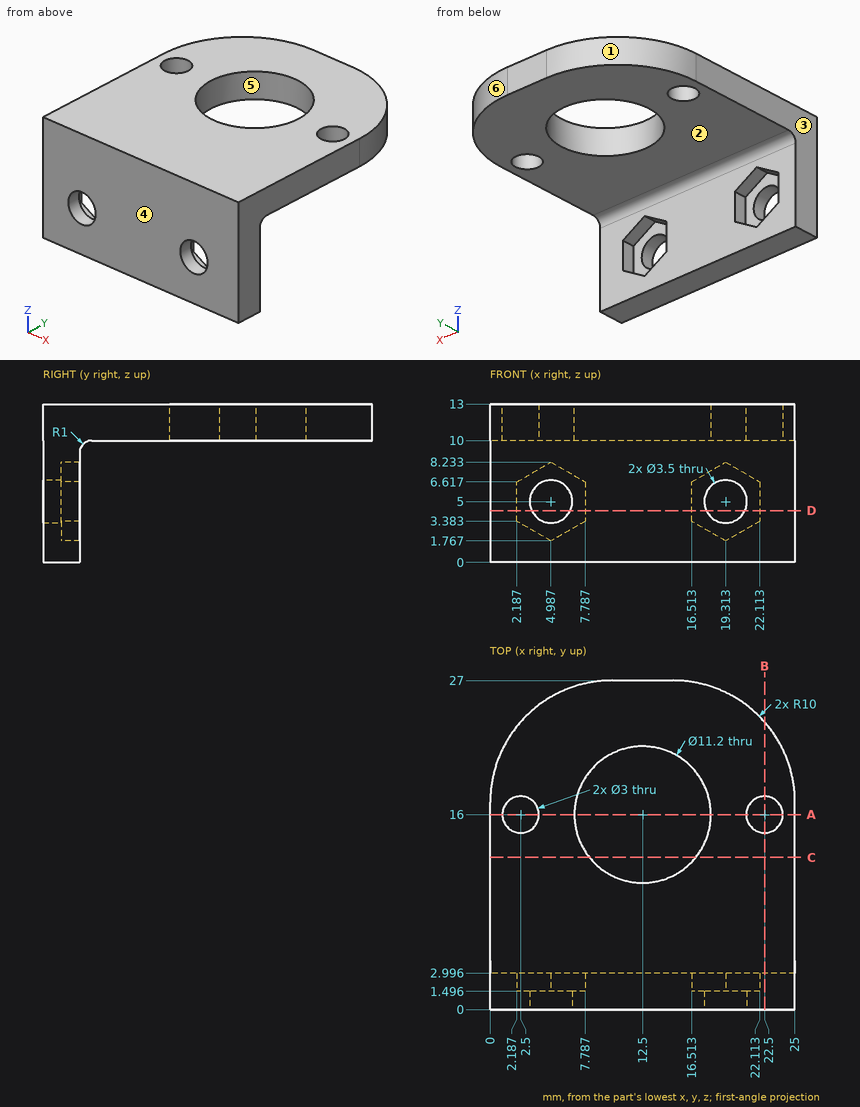
Could you check a few things on this drawing? It's one solid part, dimensions in mm from its lowest x, y, z. A direction names the side the tool comes from. Give positions to 0.01 mm unless a question says otherwise; leave off trailing zeros. Write each loop counter-clockwise with the first axis right and the second up, starting at its lowest first coordinate (ties: lowest second). Pieces come first, ordered by that corner, then holes.
(1) Imagine slicing it at B-B, the plane x = 22.5. Write out the boundary of the cut face in (y, z) (1 decimal).
Output values:
outline: (0, 0) - (3, 0) - (3, 9) arc R1 cw to (4, 10) - (14.5, 10) - (14.5, 13) - (0, 13) - close; (17.5, 10) - (23.6, 10) - (23.6, 13) - (17.5, 13) - close
(2) Imagine slicing it at A-A, the plane y = 16. Write out the boundary of the cut face in (x, z), and give its area (3 significant figures).
Output values:
outline: (0, 10) - (1, 10) - (1, 13) - (0, 13) - close; (4, 10) - (6.9, 10) - (6.9, 13) - (4, 13) - close; (18.1, 10) - (21, 10) - (21, 13) - (18.1, 13) - close; (24, 10) - (25, 10) - (25, 13) - (24, 13) - close
area: 23.4 mm2
(3) On a 3-axis mill with a long thin cutter (end or side, diameter ignored), from which of +Z, -Z, +X, -X, +Y, -Y can I reach the whole of each face in a straight line? I mean the marked faces 1 and 2. Say none if no direction works.
Output values:
face 1: +Z, -Z, -X, +Y
face 2: -Z, +X, -X, +Y
(4) Will these pins go through, and if not, where does the flat tip stop? pin 1 (1.7 mm diameter, centred on x = 18, z = 6, fed in from +Y); pin 2 (1.5 mm diameter, centred on x = 16, z = 7.5, fed in from +Y); pin 3 (3 mm diameter, centred on x = 19.31, z = 5, fed in from -Y); pin 4 (8 mm diameter, centred on x = 11, y = 14, fed in from +Z).
Output values:
pin 1: stops at y = 1.5
pin 2: stops at y = 3
pin 3: passes through
pin 4: stops at z = 13
(5) If I drill on L1, parallel to X at y = 0.8, z = 5; L2, parallel to Z at x = 3, y = 22.5; L3, parallel to Y at x = 12.5, z = 12.4, over which ranges is the centre line in solid material (lowest first)?
Output values:
L1: x = 0 to 3.24, 6.74 to 17.56, 21.06 to 25
L2: z = 10 to 13
L3: y = 0 to 10.4, 21.6 to 27
(6) Thinking about a two-plate mould opening in X: for the marked faces 3, 4, 5 and 6, which applies, pulls with the +X half, pulls with the -X half, needs draft (parallel to the pull), parting line crosses it, or undercut?
Output values:
face 3: pulls with the -X half
face 4: needs draft
face 5: undercut
face 6: pulls with the +X half
(7) Imagine slicing it at D-D, the plane z = 4.25. Write out the boundary of the cut face in (x, y) (1 decimal).
Output values:
outline: (0, 0) - (3.4, 0) - (3.4, 1.5) - (2.2, 1.5) - (2.2, 3) - (0, 3) - close; (6.6, 0) - (17.7, 0) - (17.7, 1.5) - (16.5, 1.5) - (16.5, 3) - (7.8, 3) - (7.8, 1.5) - (6.6, 1.5) - close; (20.9, 0) - (25, 0) - (25, 3) - (22.1, 3) - (22.1, 1.5) - (20.9, 1.5) - close
(8) Imagine slicing it at C-C, the plane y = 12.5. Write out the boundary of the cut face in (x, z).
Output values:
outline: (0, 10) - (8.13, 10) - (8.13, 13) - (0, 13) - close; (16.87, 10) - (25, 10) - (25, 13) - (16.87, 13) - close
